Geometry check sheet. Reference: drawing and pictorial views, mm from the part's lowest x, y, z. A direction names the side the tool comes from. Coordinates: 2 decimals unless noted, no trailing zeros. Loops run counter-clockwise (first coordinate to the right, second up) from the corner with the lowest first, then second, coordinate; pieces in that order, holes last. Notation, with made-up numbers: (-25, 12) - (6, 12) arc R23 ccw to (6, 26) - close; hole circle Ø3 at (54.5, 30). An arc over 180 degrees is marked (long way). Use a Markdown table: item, result. Add a question column.
1) Sectioned sample at A-A, the plane y = 10. Enter the section's corners in (x, z), then the cut area to 3 significant figures.
2) Tool access check on the marked faces 1, 2 and 3. Record the directions out of +Z, -Z, +X, -X, +Y, -Y that give a thin tool (end or side, any length) a straight path to the whole face; none if there is none.
3) Sectioned sample at B-B, the plane x = 13.5. Enter the section's corners in (y, z), then the cut area to 3 significant figures.
4) Go/stop test with flat-tipped pins: P1, Ø7, axis at x = 41.5, z = 8.5, coming from the +Y side; P2, Ø5, axis at y = 18, z = 14, coming from the -X side; P3, Ø6, axis at y = 5, z = 3, coming from the +X side; P4, Ø7, axis at y = 14, z = 6.5, coming from the +X side. Record where each tip stops, or that it passes through.
5) Thickness scan on line 1 (Y direction, x = 38, z = 4.5); line 2 (X direction, y = 7.5, z = 12.25). Record the ranges inside material, lowest first.
6) Sectioned sample at C-C, the plane z = 6. Enter the section's corners in (x, y), then the cut area to 3 significant figures.
7) Sectioned sample at D-D, the plane y = 1.5. Enter the section's corners in (x, z).
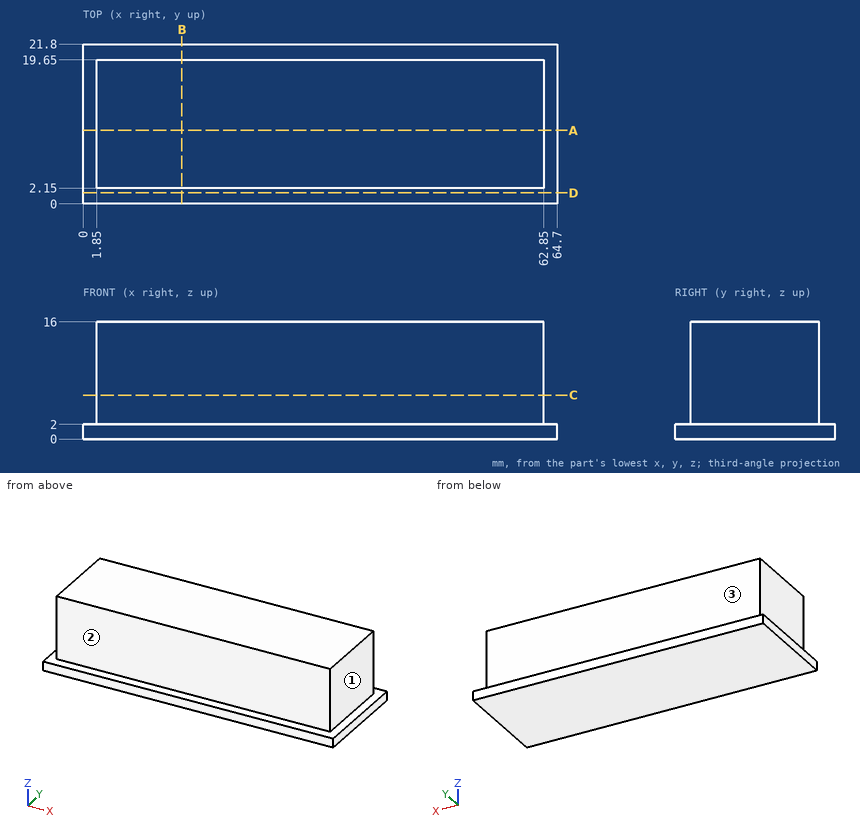
Solved:
| question | item | result |
|---|---|---|
| 1 | outline | (0, 0) - (64.7, 0) - (64.7, 2) - (62.85, 2) - (62.85, 16) - (1.85, 16) - (1.85, 2) - (0, 2) - close |
| 1 | area | 983 mm2 |
| 2 | face 1 | +Z, +X, +Y, -Y |
| 2 | face 2 | +Z, +X, -X, -Y |
| 2 | face 3 | +Z, +X, -X, +Y |
| 3 | outline | (0, 0) - (21.8, 0) - (21.8, 2) - (19.65, 2) - (19.65, 16) - (2.15, 16) - (2.15, 2) - (0, 2) - close |
| 3 | area | 289 mm2 |
| 4 | P1 | stops at y = 19.65 |
| 4 | P2 | stops at x = 1.85 |
| 4 | P3 | stops at x = 64.7 |
| 4 | P4 | stops at x = 62.85 |
| 5 | line 1 | y = 2.15 to 19.65 |
| 5 | line 2 | x = 1.85 to 62.85 |
| 6 | outline | (1.85, 2.15) - (62.85, 2.15) - (62.85, 19.65) - (1.85, 19.65) - close |
| 6 | area | 1,070 mm2 |
| 7 | outline | (0, 0) - (64.7, 0) - (64.7, 2) - (0, 2) - close |
